from build123d import *

# Parameters (mm, degrees)
CHAMFER1_SIZE           = 1
SKETCH2_R               = 11
CUT_EXTRUDE1_DEPTH      = 4
CUT_EXTRUDE2_DEPTH      = 157.004807634
CUT_EXTRUDE2_DEPTH_BACK = 157.004807634
SKETCH3_R               = 2.5


with BuildPart() as part:
    # Sketch1 → Revolve1 (revolve)
    with BuildSketch(Plane.XY, mode=Mode.PRIVATE) as revolve1_sk:
        with BuildLine():
            Line((0, 0), (0, 6.5))
            Line((0, 6.5), (1, 7.5))
            Line((1, 7.5), (13.5, 7.5))
            Line((13.5, 7.5), (13.5, 7.2))
            Line((13.5, 7.2), (15, 7.2))
            Line((15, 7.2), (15, 9))
            Line((15, 9), (49, 9))
            Line((49, 9), (50, 10))
            Line((50, 10), (61.8, 10))
            ThreePointArc((61.8, 10), (62.153553391, 10.146446609), (62.3, 10.5))
            Line((62.3, 10.5), (62.3, 12.5))
            Line((62.3, 12.5), (98, 12.5))
            Line((98, 12.5), (98, 10.5))
            ThreePointArc((98, 10.5), (98.146446609, 10.146446609), (98.5, 10))
            Line((98.5, 10), (133, 10))
            Line((133, 10), (134, 9))
            Line((134, 9), (155, 9))
            Line((155, 9), (155, 0))
            Line((155, 0), (0, 0))
        make_face()
    revolve(revolve1_sk.sketch.rotate(Axis((155, 0, 0), (-1, 0, 0)), 90), axis=Axis((155, 0, 0), (-1, 0, 0)))

    # Chamfer1
    chamfer1_edges = [part.edges().sort_by_distance(p)[0] for p in [
        (155, 0, 9),
    ]]
    chamfer(chamfer1_edges, length=CHAMFER1_SIZE)

    # Sketch2 → Cut-Extrude1 (cut, symmetric)
    with BuildSketch(Plane.XY):
        with Locations((80.15, 17.3)):
            Circle(SKETCH2_R)
    extrude(amount=CUT_EXTRUDE1_DEPTH, both=True, mode=Mode.SUBTRACT)

    # Sketch3 → Cut-Extrude2 (cut, two sides: drawn at the far end of the back side and taken through both)
    with BuildSketch(Plane(origin=(0, 0, 0), x_dir=(1, 0, 0), z_dir=(0, 1, 0)).offset(-CUT_EXTRUDE2_DEPTH_BACK)):
        with Locations(Location((7, 0, 0), (0, 0, 270))):
            Circle(SKETCH3_R)
        with Locations(Location((145.5, 0, 0), (0, 0, 270))):
            Circle(SKETCH3_R)
    extrude(amount=CUT_EXTRUDE2_DEPTH + CUT_EXTRUDE2_DEPTH_BACK, mode=Mode.SUBTRACT)


solid = part.part
The model under review builds one solid part; all positions refer to its coordinate system, in mm. A direction names the side the tool comes from. Coordinates: 2 decimals unless noted, no trailing zeros. Write each loop counter-clockwise with the first axis right and the second up, starting at its lowest first coordinate (ties: lowest second). Pieces come first, ordered by that corner, then holes. Notation, with made-up numbers: M 60,6.5 L 115,6.5 A25 cw 115,28.5 Z; hole C 77.25,-21 d3. An arc over 180 degrees is marked long. Put each result on its own line as item: value.
1) Add section B-B on y = 0. State how many separate pieces and enclosed holes the cut face has, then the cut area to 3 significant figures.
Computed:
separate pieces: 1
enclosed holes: 2
area: 3,050 mm2
2) Add section D-D on x = 7. Give the boundary of the cut face in (y, z).
Computed:
outline: M -7.07,-2.5 A7.5 ccw 7.07,-2.5 Z; M -7.07,2.5 L 7.07,2.5 A7.5 ccw Z
3) Clearance check with flat-ended pins moving along their axes: pin 1 Ø2 at (x, y) = (22, -6.5) entering from +Z; pin 2 Ø4.5 at (x, z) = (145.5, 0) entering from -Y; pin 3 Ø2 at (x, y) = (31, 5) entering from -Z; pin 4 Ø4 at (x, z) = (66.5, -3) entering from +Y. State where each tip first meets the part, or that it passes through.
Computed:
pin 1: stops at z = 7.12
pin 2: passes through
pin 3: stops at z = -8.06
pin 4: stops at y = 12.46
4) Add section A-A on x = 116. Give the boundary of the cut face in (y, z), then the cut area to 3 significant figures.
Computed:
outline: C 0,0 d20
area: 314 mm2
5) Wall thickness on probe 1 along X at (y, z) = (0.5, 0); probe 2 along X at (y, z) = (4.25, -0.5); probe 3 along Z at (x, y) = (145.5, 5): over which ranges is each line inside the solid? List them lowest first. Write a range as [from, to].
Computed:
probe 1: x = [0, 4.5], [9.5, 143], [148, 155]
probe 2: x = [0, 4.55], [9.45, 143.05], [147.95, 155]
probe 3: z = [-7.48, -2.5], [2.5, 7.48]
6) For faces 4 (the cylindrical face through (14.26, -2.16, -6.87)), 5 (the flat face through (80, 10, 4)), 6 (the cylindrical face through (116, 0, 10)), 7 (the cylindrical face through (148, 0, 0)), 8 (the cylindrical face through (56, 0, 10)), list the 3-axis set-ups (+Z, -Z, +X, -X, +Y, -Y) from which the entire face can be reached by the end or side of a thin tool; tool diameter is ignored.
Computed:
face 4: none
face 5: +Y
face 6: +X
face 7: +Y, -Y
face 8: -X
7) Draft analysis for pull direction Z (two halves, no side actions). For faces 1 (the cylindrical face through (80, 6.3, 0.1)), 2 (the cylindrical face through (80.4, -12.394, 1.627)), 3 (the flat face through (0, 0, 0)), state which applies: released by +Z, released by -Z, zero draft, split by the parting line, or undercut.
Computed:
face 1: undercut
face 2: split by the parting line
face 3: zero draft
